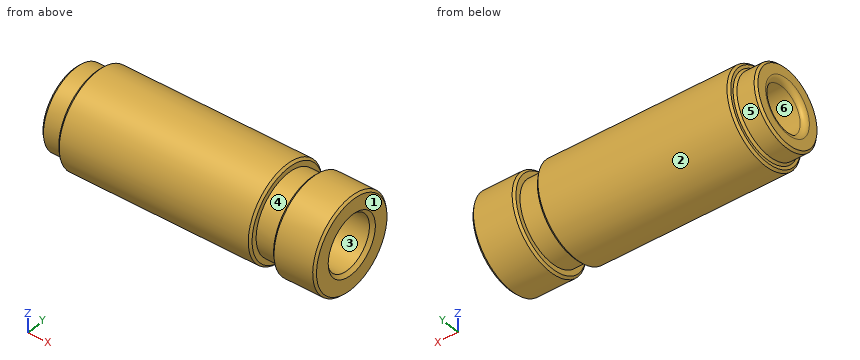
```python
from build123d import *

# Parameters (mm, degrees)
FURO_ROSCADO_DE_M14X1_51_D           = 12.5
FURO_ROSCADO_DE_M14X1_51_DEPTH       = 32
FURO_ROSCADO_DE_M14X1_51_CSINK_D     = 14.05
FURO_ROSCADO_DE_M14X1_51_CSINK_ANGLE = 90
FURO_ROSCADO_DE_M14X1_51_TIP         = 3.755378869
FURO1_D                              = 10.65
FURO1_DEPTH                          = 33
CHANFRO1_SIZE                        = 0.5
FILETE1_R                            = 1.2
CHANFRO2_SIZE                        = 0.5


with BuildPart() as part:
    # Esboço1 → Revolução1 (revolve)
    with BuildSketch(Plane.XY, mode=Mode.PRIVATE) as revolu_o1_sk:
        Polygon((0, 0), (65, 0), (65, 11), (55, 11), (55, 9.3), (50, 9.3), (50, 11), (5, 11), (5, 9.3), (0, 9.3), align=None)
    revolve(revolu_o1_sk.sketch.rotate(Axis((0, 0, 0), (1, 0, 0)), 90), axis=Axis((0, 0, 0), (1, 0, 0)))

    # Furo roscado de M14x1.51
    with Locations(Plane(origin=(65, 0, 0), x_dir=(0, 0, -1), z_dir=(1, 0, 0))):
        with Locations((0, 0)):
            CounterSinkHole(FURO_ROSCADO_DE_M14X1_51_D / 2, FURO_ROSCADO_DE_M14X1_51_CSINK_D / 2, depth=FURO_ROSCADO_DE_M14X1_51_DEPTH, counter_sink_angle=FURO_ROSCADO_DE_M14X1_51_CSINK_ANGLE)
            with Locations((0, 0, -(FURO_ROSCADO_DE_M14X1_51_DEPTH + FURO_ROSCADO_DE_M14X1_51_TIP / 2))):  # 118° drill point
                Cone(0, FURO_ROSCADO_DE_M14X1_51_D / 2, FURO_ROSCADO_DE_M14X1_51_TIP, mode=Mode.SUBTRACT)

    # Furo1
    with Locations(Plane.ZY):
        with Locations((0, 0)):
            Hole(FURO1_D / 2, depth=FURO1_DEPTH)

    # Chanfro1
    chanfro1_edges = [part.edges().sort_by_distance(p)[0] for p in [
        (5, 0, -9.3),
        (5, 0, -11),
        (50, 0, -11),
    ]]
    chamfer(chanfro1_edges, length=CHANFRO1_SIZE)

    # Filete1
    filete1_edges = [part.edges().sort_by_distance(p)[0] for p in [
        (0, 0, 5.325),
    ]]
    fillet(filete1_edges, radius=FILETE1_R)

    # Chanfro2
    chanfro2_edges = [part.edges().sort_by_distance(p)[0] for p in [
        (65, 0, -11),
        (0, 0, -9.3),
        (55, 0, -11),
    ]]
    chamfer(chanfro2_edges, length=CHANFRO2_SIZE)


solid = part.part
```
Design review of the part built by this model. Coordinates are the model's own, in mm. Face numbers are marked on the shaded views. A direction names the side the tool comes from. Give positions to 0.01 mm unless a question says otherwise; leave off trailing zeros. Write each loop counter-clockwise with the first axis right and the second up, starting at its lowest first coordinate (ties: lowest second). Pieces come first, ordered by that corner, then holes. Notation, with made-up numbers: (29, -15) - (67, -15) arc R31 cw to (67, 24) - close; hole circle Ø1 at (27.5, 60.5). An arc over 180 degrees is marked (long way). Return JSON: item names as keys, results as strings. Group by question number.
(1) To check wall thickness, follow probe 1 along Y at (x, z) = (24.5, 0) (3 decimals); probe 2 along Y at (x, z) = (54, 0); probe 3 along Z at (x, y) = (15.5, 4). State the ranges of each line that lie inside material, in increasing order.
(2) Mouldability with a two-part tool opening along Y and no side actions: class the marked faces 1, 2 and 3 as +Y half, -Y half, draft (parallel to the pull), parting line (faces both ways), or undercut.
(3) Machinability: for the marked faces 4, 5 and 6, which of the approach directions +Z, -Z, +X, -X, +Y, -Y give a long, thin tool a straight path to every point of the face, cutting with its end or side? Answer none if there is none.
(4) We need section B-B, the plane x = 34.5. Give the boundary of the cut face in (y, z), then the cut area to 3 significant figures.
(5) We need section A-A, the plane x = 23. Give the boundary of the cut face in (y, z) (3 decimals).
(6) Insertion check: pin 1 (1 mm diameter, centred on x = 31, z = 7, fed in from +Y); pin 2 (2 mm diameter, centred on y = 4.5, z = 3, fed in from -X); pin 3 (12 mm diameter, centred on x = 36, y = -8, fed in from +Z); pin 4 (7.5 mm diameter, centred on y = 0, z = 0, fed in from -X). Each pin has a flat end and moves straight along its axis. Give the tip position at first contact, or say it passes through.
Reported:
{
 "1": {"probe 1": "y = -11 to -5.325, 5.325 to 11", "probe 2": "y = -9.3 to -6.25, 6.25 to 9.3", "probe 3": "z = -10.25 to -3.52, 3.52 to 10.25"},
 "2": {"face 1": "draft", "face 2": "parting line", "face 3": "undercut"},
 "3": {"face 4": "none", "face 5": "-X", "face 6": "+X, -X"},
 "4": {"outline": "circle Ø22 at (0, 0); hole circle Ø12.5 at (0, 0)", "area": "257 mm2"},
 "5": {"outline": "circle Ø22 at (0, 0); hole circle Ø10.65 at (0, 0)"},
 "6": {"pin 1": "stops at y = 8.87", "pin 2": "stops at x = 0.01", "pin 3": "stops at z = 10.82", "pin 4": "passes through"}
}
